Autodesk Inventor part; units mm, degrees
ref_plane "YZ Plane" through (0, 0, 0) normal (1, 0, 0) x (0, 1, 0)
ref_plane "XZ Plane" through (0, 0, 0) normal (0, 1, 0) x (-1, 0, 0)
ref_plane "XY Plane" through (0, 0, 0) normal (0, 0, 1) x (1, 0, 0)
sketch "Эскиз1" plane through (0, 0, 0) normal (0, 0, 1) x (1, 0, 0)
  line L0 (0, 0) -> (32, 0)
  line L1 (0, 7) -> (32, 7)
  line L2 (4, 13.5) -> (2.5, 13.5)
  line L3 (2.5, 13.5) -> (2.1775, 10.5)
  line L4 (2.1775, 10.5) -> (1.9988, 9)
  line L5 (1.9988, 9) -> (0, 9)
  line L6 (0, 9) -> (0, 7)
  line L7 (4, 13.5) -> (4, 8.1664)
  line L8 (4, 13.5) -> (5.5, 13.5)
  line L9 (5.5, 13.5) -> (5.8225, 10.5)
  line L10 (5.8225, 10.5) -> (6.0012, 9)
  line L11 (6.0012, 9) -> (8, 9)
  line L12 (13.5, 13.5) -> (13.8225, 10.5)
  line L13 (13.8225, 10.5) -> (14.0012, 9)
  line L14 (14.0012, 9) -> (16, 9)
  line L15 (10.1775, 10.5) -> (9.9988, 9)
  line L16 (10.5, 13.5) -> (10.1775, 10.5)
  line L17 (9.9988, 9) -> (8, 9)
  line L18 (16, 9) -> (16, 13.7658)
  line L19 (28, 13.5) -> (29.5, 13.5)
  line L20 (29.5, 13.5) -> (29.8225, 10.5)
  line L21 (29.8225, 10.5) -> (30.0012, 9)
  line L22 (26.1775, 10.5) -> (25.9988, 9)
  line L23 (26.5, 13.5) -> (26.1775, 10.5)
  line L24 (28, 13.5) -> (26.5, 13.5)
  line L25 (25.9988, 9) -> (24, 9)
  line L26 (17.9988, 9) -> (16, 9)
  line L27 (18.1775, 10.5) -> (17.9988, 9)
  line L28 (18.5, 13.5) -> (18.1775, 10.5)
  line L29 (21.5, 13.5) -> (21.8225, 10.5)
  line L30 (21.8225, 10.5) -> (22.0012, 9)
  line L31 (22.0012, 9) -> (24, 9)
  line L32 (30.0012, 9) -> (32, 9)
  line L33 (32, 9) -> (32, 7)
  line L34 (10.5, 13.5) -> (13.5, 13.5)
  line L35 (18.5, 13.5) -> (21.5, 13.5)
  point P0 (1.5, 8.1664)
  dimension "d14" = 32
  dimension "d15" = 14
  dimension "d16" = 27
  dimension "d20" = 4
  dimension "d22" = 3
  dimension "d33" = 1.5
  dimension "d35" = 2
  dimension "d37" = 32
revolve "Вращение1" add sketch "Эскиз1" angle 360 about axis through (0, 0, 0) along (1, 0, 0)
properties part number "Демфер пальца" material "Резина"
Input: part model. Units: mm. Frame: model coordinates. A direction names the side the tool comes from. Give positions to 0.01 mm unless a question says otherwise; leave off trailing zeros. Write each loop counter-clockwise with the first axis right and the second up, starting at its lowest first coordinate (ties: lowest second). Pieces come first, ordered by that corner, then holes.
Q1. Material intervals for probe 1 along X at (y, z) = (9, -4.5); probe 2 along Z at (x, y) = (13, 0); probe 3 along Z at (x, y) = (15, 0), sorted ascending.
Q2. Section A-A, the plane x = 19.5. Output: boundary loops of the cut face in (y, z).
Q3. Pull-direction query (X, two-part tool) for faces 1 (the face through (31.015, -1.172, 8.923)), 2 (the face through (0, 0, -7.3)), 3 (the face through (23.972, -1.172, -8.923)); classes: pulls with the +X half, pulls with the -X half, needs draft (parallel to the pull), parting line crosses it, or undercut.
Q4. First-contact query: P1, Ø10, axis at x = 7, z = 5.5, coming from the -Y side; P2, Ø1.5, axis at y = -9, z = -6.5, coming from the +X side; P3, Ø8, axis at x = 7.5, z = 6.5, coming from the -Y side. Flat tips, straight axial feed; report the tip coordinate or a pass-through.
Q5. Section B-B, the plane x = 25.5. Output: boundary loops of the cut face in (y, z), plus the area to 3 significant figures.
Q6. Set-up query: faces 4 (the face through (3.98, -2.93, 13.18)), 5 (the face through (0.985, -1.172, -8.923)), 6 (the face through (5.802, -2.317, 10.434)). Return all of +Z, -Z, +X, -X, +Y, -Y with unobstructed straight access to the full face (end or side cutting, diameter ignored); none if empty.
Filled in:
1. probe 1: x = 2.13 to 5.87, 10.13 to 13.87, 18.13 to 21.87, 26.13 to 29.87
1. probe 2: z = -13.5 to -7, 7 to 13.5
1. probe 3: z = -9 to -7, 7 to 9
2. outline: circle Ø27 at (0, 0); hole circle Ø14 at (0, 0)
3. face 1: needs draft
3. face 2: pulls with the -X half
3. face 3: undercut
4. P1: stops at y = -13.48
4. P2: stops at x = 29.84
4. P3: stops at y = -13.15
5. outline: circle Ø18 at (0, 0); hole circle Ø14 at (0, 0)
5. area: 101 mm2
6. face 4: +X, -X
6. face 5: -X
6. face 6: none
